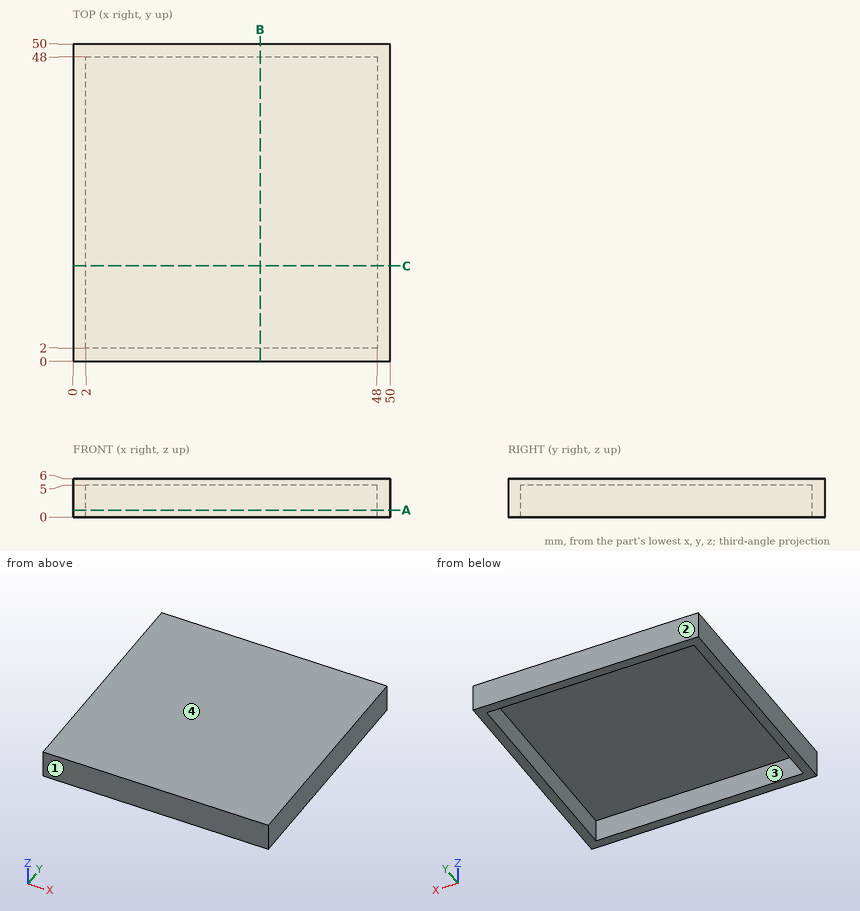
Drawing for the job (mm, zero at the part's lowest x, y, z). Give positions to 0.01 mm unless a question says otherwise; leave off trailing zeros. Order: outer loops, then holes, each group sorted by start corner. A loop starts at its lowest first (then second) coordinate and runs counter-clockwise, first axis right, second up. Notation, with made-up numbers: M 46,25 L 51,25 A11 ccw 51,35 Z; hole C 29.5,49.25 d6. An arc over 180 degrees is marked long. Put each result on its own line as item: value.
Item 1: Slice it at A-A, the plane z = 1.1. Write the cut outline in (x, y), plus the area to 3 significant figures.
From the geometry:
outline: M 0,0 L 50,0 L 50,50 L 0,50 Z; hole M 2,2 L 48,2 L 48,48 L 2,48 Z
area: 384 mm2
Item 2: Two-plate mould, pull along Y, no slides. Class the marked faces 1, 2, 3 and 4: +Y half, -Y half, draft (parallel to the pull), parting line (faces both ways), or undercut.
From the geometry:
face 1: -Y half
face 2: +Y half
face 3: undercut
face 4: draft
Item 3: Probe line 1 (X direction, y = 15.5, z = 4.55); line 2 (Z direction, x = 40, y = 20). List the from-to ranges inside material, lowest first. Write a range as [from, to].
From the geometry:
line 1: x = [0, 2], [48, 50]
line 2: z = [5, 6]
Item 4: Flat gauge pin, fed straight in: pin 1 Ø2 at (x, y) = (29.5, 13.5) entering from -Z. Where does the tip first touch, or does it go through?
From the geometry:
pin 1: stops at z = 5
Item 5: Slice it at B-B, the plane x = 29.5. Write the cut outline in (y, z).
From the geometry:
outline: M 0,0 L 2,0 L 2,5 L 48,5 L 48,0 L 50,0 L 50,6 L 0,6 Z
